```python
from build123d import *

# Parameters (mm, degrees)
SKETCH1_W           = 55.1
SKETCH1_H           = 27.49
BOSS_EXTRUDE1_DEPTH = 1
FILLET2_R           = 0.5
SKETCH3_W           = 59.1
SKETCH3_H           = 31.49
SKETCH3_W_2         = 57.1
SKETCH3_H_2         = 29.49
BOSS_EXTRUDE2_DEPTH = 2


with BuildPart() as part:
    # Sketch1 → Boss-Extrude1 (new body)
    with BuildSketch(Plane.XY):
        with BuildLine():
            Line((-28.55, 16.745), (28.55, 16.745))
            ThreePointArc((28.55, 16.745), (29.964213562, 16.159213562), (30.55, 14.745))
            Line((30.55, 14.745), (30.55, -14.745))
            ThreePointArc((30.55, -14.745), (29.964213562, -16.159213562), (28.55, -16.745))
            Line((28.55, -16.745), (-28.55, -16.745))
            ThreePointArc((-28.55, -16.745), (-29.964213562, -16.159213562), (-30.55, -14.745))
            Line((-30.55, -14.745), (-30.55, 14.745))
            ThreePointArc((-30.55, 14.745), (-29.964213562, 16.159213562), (-28.55, 16.745))
        make_face()
        Rectangle(SKETCH1_W, SKETCH1_H, mode=Mode.SUBTRACT)
    extrude(amount=BOSS_EXTRUDE1_DEPTH)

    # Fillet2
    fillet2_edges = [part.edges().sort_by_distance(p)[0] for p in [
        (0, 16.745, 0),
        (29.964213562, 16.159213562, 0),
        (30.55, 0, 0),
        (29.964213562, -16.159213562, 0),
        (27.55, 0, 0),
        (0, 13.745, 0),
        (-27.55, 0, 0),
        (0, -13.745, 0),
        (0, -16.745, 0),
        (-29.964213562, -16.159213562, 0),
        (-30.55, 0, 0),
        (-29.964213562, 16.159213562, 0),
    ]]
    fillet(fillet2_edges, radius=FILLET2_R)

    # Sketch3 → Boss-Extrude2 (add)
    with BuildSketch(Plane.XY.offset(1)):
        Rectangle(SKETCH3_W, SKETCH3_H)
        Rectangle(SKETCH3_W_2, SKETCH3_H_2, mode=Mode.SUBTRACT)
    extrude(amount=BOSS_EXTRUDE2_DEPTH)


solid = part.part
```
Check sheet for the modelled part. Datum: model origin and axes. Units: mm. A direction names the side the tool comes from. Round coordinates to 2 decimals unless told otherwise and drop trailing zeros. Write each loop counter-clockwise with the first axis right and the second up, starting at its lowest first coordinate (ties: lowest second). Pieces come first, ordered by that corner, then holes. Notation, with made-up numbers: (-15.5, 33.5) -> (16.5, 33.5) arc R8 cw to (16.5, 46.5) -> close; hole circle Ø10 at (-28, 17). An arc over 180 degrees is marked (long way). Put each result on its own line as item: value.
(1) Sectioned sample at C-C (x = -11.5). Enter the section's corners in (y, z) (3 decimals), plus the area to 3 significant figures.
Values found:
outline: (-16.745, 0.5) arc R0.5 ccw to (-16.245, 0) -> (-14.245, 0) arc R0.5 ccw to (-13.745, 0.5) -> (-13.745, 1) -> (-14.745, 1) -> (-14.745, 3) -> (-15.745, 3) -> (-15.745, 1) -> (-16.745, 1) -> close; (13.745, 0.5) arc R0.5 ccw to (14.245, 0) -> (16.245, 0) arc R0.5 ccw to (16.745, 0.5) -> (16.745, 1) -> (15.745, 1) -> (15.745, 3) -> (14.745, 3) -> (14.745, 1) -> (13.745, 1) -> close
area: 9.79 mm^2
(2) Go/stop test with flat-tipped pins: pin 1 Ø1.6 at (x, z) = (-6, 2) entering from -Y (3 decimals); pin 2 Ø1.6 at (y, z) = (2.5, 1.5) entering from +X; pin 3 Ø1.6 at (y, z) = (2, 2.5) entering from -X; pin 4 Ø0.6 at (x, z) = (11, 2) entering from +Y (3 decimals). Record where each tip stops, or that it passes through.
Values found:
pin 1: stops at y = -15.745
pin 2: stops at x = 30.55
pin 3: stops at x = -29.55
pin 4: stops at y = 15.745
(3) Tool access check on faces 5 (the face through (29.55, 0, 2)), 6 (the face through (28.55, 0, 2)), 7 (the face through (-29.55, 0, 2)), 8 (the face through (0, 15.745, 2)). Record the directions out of +Z, -Z, +X, -X, +Y, -Y that give a thin tool (end or side, any length) a straight path to the whole face; none if there is none.
Values found:
face 5: +Z, +X, +Y, -Y
face 6: +Z
face 7: +Z, -X, +Y, -Y
face 8: +Z, +X, -X, +Y
(4) Sectioned sample at B-B (z = 2.15). Enter the section's corners in (x, y) (3 decimals), plus the area to 3 significant figures.
Values found:
outline: (-29.55, -15.745) -> (29.55, -15.745) -> (29.55, 15.745) -> (-29.55, 15.745) -> close; hole (-28.55, -14.745) -> (28.55, -14.745) -> (28.55, 14.745) -> (-28.55, 14.745) -> close
area: 177 mm^2
(5) Sectioned sample at A-A (y = -9). Enter the section's corners in (x, z).
Values found:
outline: (-30.55, 0.5) arc R0.5 ccw to (-30.05, 0) -> (-28.05, 0) arc R0.5 ccw to (-27.55, 0.5) -> (-27.55, 1) -> (-28.55, 1) -> (-28.55, 3) -> (-29.55, 3) -> (-29.55, 1) -> (-30.55, 1) -> close; (27.55, 0.5) arc R0.5 ccw to (28.05, 0) -> (30.05, 0) arc R0.5 ccw to (30.55, 0.5) -> (30.55, 1) -> (29.55, 1) -> (29.55, 3) -> (28.55, 3) -> (28.55, 1) -> (27.55, 1) -> close
(6) Mould release check, pull along Y, two halves, no side actions. Record for faces 1 (the face through (9, -16, 1)), 2 (the face through (0, 14.745, 2)), 3 (the face through (-29.98, 16.144, 0.746)), 4 (the face through (0, -15.745, 2)): released by +Y, released by -Y, zero draft, split by the parting line, or undercut.
Values found:
face 1: zero draft
face 2: undercut
face 3: released by +Y
face 4: released by -Y
(7) Material ranges on line 1 (X direction, y = 8, z = 2.35); line 2 (Y direction, x = 6, z = 1.05) (3 decimals); line 3 (X direction, y = 6, z = 0.8), recorded low to high.
Values found:
line 1: x = -29.55 to -28.55, 28.55 to 29.55
line 2: y = -15.745 to -14.745, 14.745 to 15.745
line 3: x = -30.55 to -27.55, 27.55 to 30.55
